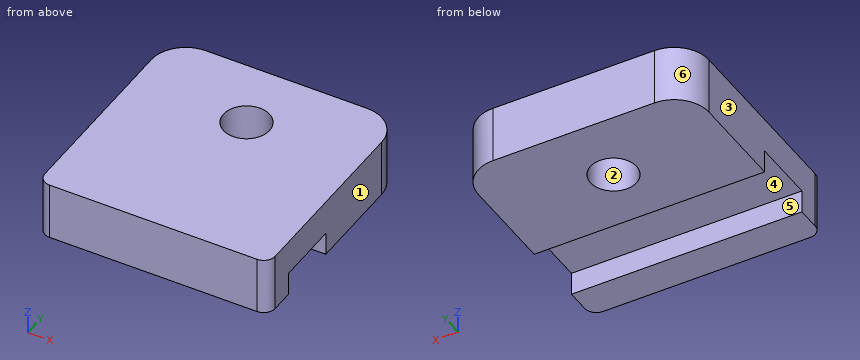
from build123d import *

# Parameters (mm, degrees)
SKETCH1_W           = 20
SKETCH1_H           = 20
BOSS_EXTRUDE1_DEPTH = 5
SKETCH2_R           = 2
CUT_EXTRUDE1_DEPTH  = 6
FILLET1_R           = 3
FILLET2_R           = 1
SKETCH3_W           = 20
SKETCH3_H           = 5.6
CUT_EXTRUDE2_DEPTH  = 2


with BuildPart() as part:
    # Sketch1 → Boss-Extrude1 (new body)
    with BuildSketch(Plane.XY):
        Rectangle(SKETCH1_W, SKETCH1_H)
    extrude(amount=BOSS_EXTRUDE1_DEPTH)

    # Sketch2 → Cut-Extrude1 (cut, through all)
    with BuildSketch(Plane.XY.offset(5)):
        with Locations((0, 4)):
            Circle(SKETCH2_R)
    extrude(amount=-CUT_EXTRUDE1_DEPTH, mode=Mode.SUBTRACT)

    # Fillet1
    fillet1_edges = [part.edges().sort_by_distance(p)[0] for p in [
        (-10, 10, 2.5),
        (10, 10, 2.5),
    ]]
    fillet(fillet1_edges, radius=FILLET1_R)

    # Fillet2
    fillet2_edges = [part.edges().sort_by_distance(p)[0] for p in [
        (10, -10, 2.5),
        (-10, -10, 2.5),
    ]]
    fillet(fillet2_edges, radius=FILLET2_R)

    # Sketch3 → Cut-Extrude2 (cut)
    with BuildSketch(Plane(origin=(0, 0, 0), x_dir=(-1, 0, 0), z_dir=(0, 0, -1))):
        with Locations((0, -4.2)):
            Rectangle(SKETCH3_W, SKETCH3_H)
    extrude(amount=-CUT_EXTRUDE2_DEPTH, mode=Mode.SUBTRACT)


solid = part.part
Can you work these out from the model? Positions are in its coordinate system, mm. Face numbers are marked on the shaded views. A direction names the side the tool comes from. Coordinates: 2 decimals unless noted, no trailing zeros. Loops run counter-clockwise (first coordinate to the right, second up) from the corner with the lowest first, then second, coordinate; pieces in that order, holes last. Notation, with made-up numbers: M 44,-38.75 L 51,-38.75 A11 cw 51,-34.75 Z; hole C -24.75,37.5 d3. An arc over 180 degrees is marked long. Return JSON: item names as keys, results as strings. Group by question number.
Item 1: Imagine slicing it at C-C (z = 4). Please give me the cut outline in (x, y), and give its area (3 significant figures).
Item 2: If I drill on L1, parallel to Y at x = 0, z = 1.55; L2, parallel to Y at x = -3.5, z = 1.9; L3, parallel to Y at x = 0, z = 3.2, over which ranges is the centre line in solid material (lowest first)? Write a range as from..to.
Item 3: Imagine slicing it at D-D (x = 0). Please give me the cut outline in (y, z).
Item 4: Thinking about a two-plate mould opening in X: for the marked faces 1, 2, 3 and 4, which applies, released by +X, released by -X, zero draft, split by the parting line, or undercut?
Item 5: Imagine slicing it at B-B (y = 4.75). Please give me the cut outline in (x, z).
Item 6: On a 3-axis mill with a long thin cutter (end or side, diameter ignored), from which of +Z, -Z, +X, -X, +Y, -Y can I reach the whole of each face in a straight line? I mean the marked faces 5 and 6. Say none if no direction works.
Item 7: Imagine slicing it at A-A (z = 0.8). Please give me the cut outline in (x, y).
Verdict:
{
 "1": {"outline": "M -10,-9 A1 ccw -9,-10 L 9,-10 A1 ccw 10,-9 L 10,7 A3 ccw 7,10 L -7,10 A3 ccw -10,7 Z; hole C 0,4 d4", "area": "383 mm^2"},
 "2": {"L1": "y = -10..-7, -1.4..2, 6..10", "L2": "y = -10..-7, -1.4..10", "L3": "y = -10..2, 6..10"},
 "3": {"outline": "M -10,0 L -7,0 L -7,2 L -1.4,2 L -1.4,0 L 2,0 L 2,5 L -10,5 Z; M 6,0 L 10,0 L 10,5 L 6,5 Z"},
 "4": {"face 1": "released by +X", "face 2": "undercut", "face 3": "released by -X", "face 4": "zero draft"},
 "5": {"outline": "M -10,0 L -1.85,0 L -1.85,5 L -10,5 Z; M 1.85,0 L 10,0 L 10,5 L 1.85,5 Z"},
 "6": {"face 5": "-Z, +X, -X", "face 6": "+Z, -Z, -X, +Y"},
 "7": {"outline": "M -10,-9 A1 ccw -9,-10 L 9,-10 A1 ccw 10,-9 L 10,-7 L -10,-7 Z; M -10,-1.4 L 10,-1.4 L 10,7 A3 ccw 7,10 L -7,10 A3 ccw -10,7 Z; hole C 0,4 d4"}
}
